from build123d import *

# Parameters (mm, degrees)
SKETCH1_W           = 190.5
SKETCH1_H           = 190.5
BOSS_EXTRUDE1_DEPTH = 3.175
SKETCH4_W           = 20.902
SKETCH4_H           = 18.5208
SKETCH4_W_2         = 18.9176
SKETCH4_W_3         = 58.3406
SKETCH4_W_4         = 41.3228
SKETCH4_H_2         = 18.521
SKETCH4_W_5         = 31.0406
SKETCH4_H_3         = 19.0502
SKETCH4_W_6         = 19.6834
SKETCH4_W_7         = 16.801
SKETCH4_W_8         = 17.3964
SKETCH4_W_9         = 69.9784
SKETCH4_H_4         = 21.4674
SKETCH4_W_10        = 9.1858
SKETCH4_H_5         = 19.05
SKETCH4_W_11        = 40.0886
SKETCH4_W_12        = 16.9334
SKETCH4_W_13        = 18.124
SKETCH4_W_14        = 28.07
SKETCH4_W_15        = 31.7698
SKETCH4_W_16        = 50.5814
SKETCH4_H_6         = 20.1082
SKETCH4_W_17        = 27.3424
SKETCH4_W_18        = 8.028
SKETCH4_W_19        = 39.4186
SKETCH4_W_20        = 17.8594
SKETCH4_W_21        = 30.497
SKETCH4_H_7         = 20.1084
SKETCH4_W_22        = 18.3882
SKETCH4_W_23        = 46.8316
SKETCH4_W_24        = 8.6652
SKETCH4_W_25        = 50.754
SKETCH4_W_26        = 40.3286
SKETCH4_H_8         = 20.3728
SKETCH4_W_27        = 8.202
SKETCH4_W_28        = 7.8052
SKETCH4_W_29        = 17.198
SKETCH4_W_30        = 7.5406
SKETCH4_W_31        = 49.5384
SKETCH4_W_32        = 59.9076
SKETCH4_W_33        = 9.6572
SKETCH4_W_34        = 50.861
CUT_EXTRUDE2_DEPTH  = 4.175


with BuildPart() as part:
    # Sketch1 → Boss-Extrude1 (new body)
    with BuildSketch(Plane(origin=(0, 0, 0), x_dir=(1, 0, 0), z_dir=(0, 1, 0))):
        Rectangle(SKETCH1_W, SKETCH1_H)
    extrude(amount=BOSS_EXTRUDE1_DEPTH)

    # Sketch4 → Cut-Extrude2 (cut, through all)
    with BuildSketch(Plane(origin=(0, 3.175, 0), x_dir=(1, 0, 0), z_dir=(0, 1, 0))):
        with Locations((-75.0878, 75.8609)):
            Rectangle(SKETCH4_W, SKETCH4_H)
        with Locations((-44.6608, 75.8609)):
            Rectangle(SKETCH4_W_2, SKETCH4_H)
        with Locations((4.9001, 75.8609)):
            Rectangle(SKETCH4_W_3, SKETCH4_H)
        with Locations((64.7206, 75.8608)):
            Rectangle(SKETCH4_W_4, SKETCH4_H_2)
        with Locations((-70.0185, 50.9899)):
            Rectangle(SKETCH4_W_5, SKETCH4_H_3)
        with Locations((-34.8388, 50.9899)):
            Rectangle(SKETCH4_W_6, SKETCH4_H_3)
        with Locations((-14.6268, 50.9899)):
            Rectangle(SKETCH4_W_7, SKETCH4_H_3)
        with Locations((4.721, 50.9899)):
            Rectangle(SKETCH4_W_8, SKETCH4_H_3)
        with Locations((50.3928, 49.7813)):
            Rectangle(SKETCH4_W_9, SKETCH4_H_4)
        with Locations((39.2539, 25.3254)):
            Rectangle(SKETCH4_W_10, SKETCH4_H_5)
        with Locations((-65.4945, 25.3254)):
            Rectangle(SKETCH4_W_11, SKETCH4_H_5)
        with Locations((-34.7345, 25.3254)):
            Rectangle(SKETCH4_W_12, SKETCH4_H_5)
        with Locations((-14.6923, 25.3254)):
            Rectangle(SKETCH4_W_13, SKETCH4_H_5)
        with Locations((18.9639, 25.3254)):
            Rectangle(SKETCH4_W_14, SKETCH4_H_5)
        with Locations((69.4971, 25.3254)):
            Rectangle(SKETCH4_W_15, SKETCH4_H_5)
        with Locations((-60.2481, 0.19)):
            Rectangle(SKETCH4_W_16, SKETCH4_H_6)
        with Locations((-0.2517, 0.19)):
            Rectangle(SKETCH4_W_17, SKETCH4_H_6)
        with Locations((19.4598, 0.19)):
            Rectangle(SKETCH4_W_18, SKETCH4_H_6)
        with Locations((65.6727, 0.19)):
            Rectangle(SKETCH4_W_19, SKETCH4_H_6)
        with Locations((34.2556, 0.19)):
            Rectangle(SKETCH4_W_20, SKETCH4_H_6)
        with Locations((-70.2903, -24.9455)):
            Rectangle(SKETCH4_W_21, SKETCH4_H_7)
        with Locations((-44.2841, -24.9455)):
            Rectangle(SKETCH4_W_22, SKETCH4_H_7)
        with Locations((-9.93, -24.9455)):
            Rectangle(SKETCH4_W_23, SKETCH4_H_7)
        with Locations((19.5051, -24.9455)):
            Rectangle(SKETCH4_W_24, SKETCH4_H_7)
        with Locations((60.0051, -24.9455)):
            Rectangle(SKETCH4_W_25, SKETCH4_H_7)
        with Locations((-65.3745, -50.2132)):
            Rectangle(SKETCH4_W_26, SKETCH4_H_8)
        with Locations((-29.7731, -50.2132)):
            Rectangle(SKETCH4_W_27, SKETCH4_H_8)
        with Locations((-4.7699, -50.2132)):
            Rectangle(SKETCH4_W_12, SKETCH4_H_8)
        with Locations((-19.9173, -50.2132)):
            Rectangle(SKETCH4_W_28, SKETCH4_H_8)
        with Locations((14.8093, -50.2132)):
            Rectangle(SKETCH4_W_29, SKETCH4_H_8)
        with Locations((29.4275, -50.2132)):
            Rectangle(SKETCH4_W_30, SKETCH4_H_8)
        with Locations((60.6129, -50.2132)):
            Rectangle(SKETCH4_W_31, SKETCH4_H_8)
        with Locations((-55.585, -75.6132)):
            Rectangle(SKETCH4_W_32, SKETCH4_H_8)
        with Locations((-0.1649, -75.6132)):
            Rectangle(SKETCH4_W_33, SKETCH4_H_8)
        with Locations((59.9515, -75.6132)):
            Rectangle(SKETCH4_W_34, SKETCH4_H_8)
    extrude(amount=-CUT_EXTRUDE2_DEPTH, mode=Mode.SUBTRACT)


solid = part.part
Read the model definition and answer for the solid it produces. Units are mm, in the model's axes. Give positions to 0.01 mm unless a question says otherwise; leave off trailing zeros. Use CSV: the item, a comma, the result in double quotes. Start each with the question number.
Item 1: Consider line 1 (Z direction, x = -26, y = 1.1) (3 decimals); line 2 (X direction, y = 2.8, z = -50); line 3 (X direction, y = 1.9, z = 3.5). Determine where each line is inside the solid, lowest interval first.
Item 2: Flat-ended cylindrical pins translate along their axes: P1, Ø1.5, axis at x = -11.5, z = 2.5, coming from the +Y side; P2, Ø2, axis at x = 3.5, z = -27, coming from the -Y side. Find the tip coordinate at first contact, or state that the pin passes through.
Item 3: The part is cut by section A-A, the plane x = 10.5. Count the separate pieces of the cut face and the enclosed holes in it, and give its area (3 significant figures).
Taken from the geometry:
1,line 1,"-95.25 to -60.515, -41.465 to 14.891, 35 to 40.027, 60.4 to 65.427, 85.8 to 95.25"
1,line 2,"-95.25 to -85.54, -54.5 to -44.68, -25 to -23.03, -6.23 to -3.98, 13.42 to 15.4, 85.38 to 95.25"
1,line 3,"-95.25 to -85.54, -34.96 to -13.92, 13.42 to 15.45, 23.47 to 25.33, 43.19 to 45.96, 85.38 to 95.25"
2,P1,"through"
2,P2,"y = 0"
3,separate pieces,"7"
3,enclosed holes,"0"
3,area,"233 mm2"
